from build123d import *

# Parameters (mm, degrees)
SKETCH_R      = 64
SKETCH_R_2    = 2.1
SKETCH_R_3    = 33.5
PAD_DEPTH     = 3
SKETCH001_R   = 37.5
SKETCH001_R_2 = 33.5
PAD001_DEPTH  = 17
SKETCH002_R   = 40.5
SKETCH002_R_2 = 37.5
PAD002_DEPTH  = 6
CHAMFER_SIZE  = 0.5


with BuildPart() as part:
    # Sketch → Pad (new body)
    with BuildSketch(Plane.XY):
        Circle(SKETCH_R)
        with Locations((-28.25, 48.930435)):
            Circle(SKETCH_R_2, mode=Mode.SUBTRACT)
        with Locations((28.25, 48.930435)):
            Circle(SKETCH_R_2, mode=Mode.SUBTRACT)
        with Locations((56.5, 0)):
            Circle(SKETCH_R_2, mode=Mode.SUBTRACT)
        with Locations((28.25, -48.930435)):
            Circle(SKETCH_R_2, mode=Mode.SUBTRACT)
        with Locations((-28.25, -48.930435)):
            Circle(SKETCH_R_2, mode=Mode.SUBTRACT)
        with Locations((-56.5, 0)):
            Circle(SKETCH_R_2, mode=Mode.SUBTRACT)
        Circle(SKETCH_R_3, mode=Mode.SUBTRACT)
    extrude(amount=PAD_DEPTH)

    # Sketch001 (on Face10 of Pad) → Pad001 (join)
    with BuildSketch(Plane.XY.offset(3)):
        Circle(SKETCH001_R)
        Circle(SKETCH001_R_2, mode=Mode.SUBTRACT)
    extrude(amount=PAD001_DEPTH)

    # Sketch002 (on Face3 of Pad001) → Pad002 (join)
    with BuildSketch(Plane.XY.offset(3)):
        Circle(SKETCH002_R)
        Circle(SKETCH002_R_2, mode=Mode.SUBTRACT)
    extrude(amount=PAD002_DEPTH)

    # Chamfer
    chamfer_edges = [part.edges().sort_by_distance(p)[0] for p in [
        (-37.5, 0, 20),
    ]]
    chamfer(chamfer_edges, length=CHAMFER_SIZE)


solid = part.part
Could you check a few things on this model? Use its own coordinates, in mm. A direction names the side the tool comes from. Give positions to 0.01 mm unless a question says otherwise; leave off trailing zeros. Order: outer loops, then holes, each group sorted by start corner. A loop starts at its lowest first (then second) coordinate and runs counter-clockwise, first axis right, second up. Notation, with made-up numbers: (-31, -32) -> (-9, -32) arc R25 cw to (-9, 4) -> close; hole circle Ø9 at (28, 50). An arc over 180 degrees is marked (long way). Return JSON: item names as keys, results as strings.
1. For pin 1 Ø1 at (y, z) = (-46.5, 3) entering from -X; pin 2 Ø5 at (x, y) = (-28.25, 48.93) entering from +Z; pin 3 Ø8 at (x, z) = (-26.5, 9.5) entering from -Y, each with a flat end and sliding along its axis, tell me the tip position at first contact or that it passes through.
Answer list:
{"pin 1": "stops at x = -44.5", "pin 2": "stops at z = 3", "pin 3": "stops at y = -33.65"}
2. Thinking about a two-plate mould opening in Y: for faces 3 (the flat face through (-19, 28, 20)), 4 (the cylindrical face through (58.44, -0.8, 1.48)), 5 (the cylindrical face through (-4.88, 37.18, 14.18)), 6 (the cylindrical face through (-7.262, -32.703, 9.86)), which applies, pulls with the +Y half, pulls with the -Y half, needs draft (parallel to the pull), parting line crosses it, or undercut?
Answer list:
{"face 3": "needs draft", "face 4": "undercut", "face 5": "parting line crosses it", "face 6": "undercut"}
3. I need wall thicknesses on line 1 (Y direction, x = -28.25, z = 1.1); line 2 (Z direction, x = 49, y = -35.5); line 3 (X direction, y = -2.5, z = 12.75). Which ranges of each line are inside material? Lowest first, please. Write a range as from..to.
Answer list:
{"line 1": "y = -57.43..-51.03, -46.83..-18.01, 18.01..46.83, 51.03..57.43", "line 2": "z = 0..3", "line 3": "x = -37.42..-33.41, 33.41..37.42"}
4. Imagine slicing it at D-D on x = 56.5. List the corners of the cut face in (y, z) for me.
Answer list:
{"outline": "(-30.06, 0) -> (-2.1, 0) -> (-2.1, 3) -> (-30.06, 3) -> close; (2.1, 0) -> (30.06, 0) -> (30.06, 3) -> (2.1, 3) -> close"}
5. Imagine slicing it at B-B on y = 0. List the corners of the cut face in (x, z) for me.
Answer list:
{"outline": "(-64, 0) -> (-58.6, 0) -> (-58.6, 3) -> (-64, 3) -> close; (-54.4, 0) -> (-33.5, 0) -> (-33.5, 20) -> (-37, 20) -> (-37.5, 19.5) -> (-37.5, 9) -> (-40.5, 9) -> (-40.5, 3) -> (-54.4, 3) -> close; (33.5, 0) -> (54.4, 0) -> (54.4, 3) -> (40.5, 3) -> (40.5, 9) -> (37.5, 9) -> (37.5, 19.5) -> (37, 20) -> (33.5, 20) -> close; (58.6, 0) -> (64, 0) -> (64, 3) -> (58.6, 3) -> close"}
6. On a 3-axis mill with a long thin cutter (end or side, diameter ignored), from which of +Z, -Z, +X, -X, +Y, -Y can I reach the whole of each face in a straight line? I mean faces 1 (the flat face through (28, -28, 0)), 2 (the cylindrical face through (21.77, 34.15, 5.96)). Say none if no direction works.
Answer list:
{"face 1": "-Z, +X, -X, +Y, -Y", "face 2": "+Z"}
7. Imagine slicing it at A-A on x = 0. List the corners of the cut face in (y, z) for me, then the cut area to 3 significant figures.
Answer list:
{"outline": "(-64, 0) -> (-33.5, 0) -> (-33.5, 20) -> (-37, 20) -> (-37.5, 19.5) -> (-37.5, 9) -> (-40.5, 9) -> (-40.5, 3) -> (-64, 3) -> close; (33.5, 0) -> (64, 0) -> (64, 3) -> (40.5, 3) -> (40.5, 9) -> (37.5, 9) -> (37.5, 19.5) -> (37, 20) -> (33.5, 20) -> close", "area": "355 mm2"}
8. Imagine slicing it at C-C on z = 7. List the corners of the cut face in (x, y) for me.
Answer list:
{"outline": "circle Ø81 at (0, 0); hole circle Ø67 at (0, 0)"}
